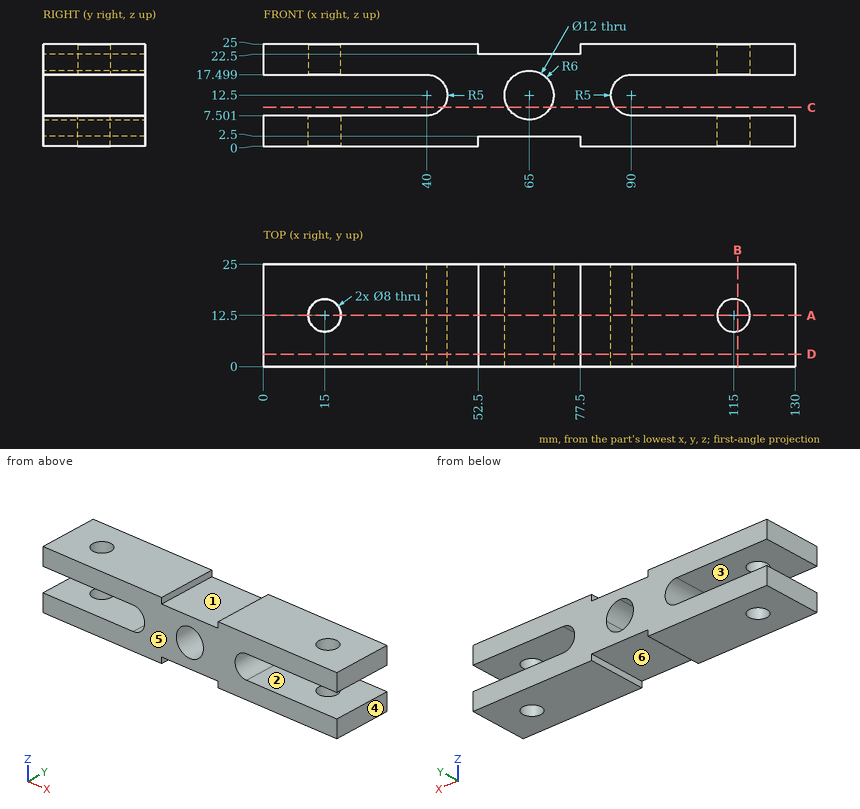
The drawing under review shows one solid part. Ordinate dimensions are in mm from its lowest x, y, z. A direction names the side the tool comes from. Coordinates: 2 decimals unless noted, no trailing zeros. Order: outer loops, then holes, each group sorted by start corner. A loop starts at its lowest first (then second) coordinate and runs counter-clockwise, first axis right, second up. Notation, with made-up numbers: (-2, 60.25) -> (4, 60.25) arc R36 cw to (4, 94.25) -> close; hole circle Ø7 at (45, 56). An arc over 180 degrees is marked (long way). Use CSV: the item, a comma, the result in double quotes. Start each with the question number.
Item 1: We need section D-D, the plane y = 3. Give the boundary of the cut face in (x, z) (1 decimal), then the cut area to 3 significant figures.
Item 2: Draft analysis for pull direction X (two halves, no side actions). For the marked faces 4, 5 and 6, state which applies: pulls with the +X half, pulls with the -X half, needs draft (parallel to the pull), parting line crosses it, or undercut.
Item 3: We need section C-C, the plane z = 9.5. Give the boundary of the cut face in (x, y).
Item 4: For the marked faces 1, 2 and 3, list the 3-axis set-ups (+Z, -Z, +X, -X, +Y, -Y) from which the entire face can be reached by the end or side of a thin tool; tool diameter is ignored.
Item 5: We need section A-A, the plane y = 12.5. Give the number of separate pieces and of enclosed holes in the cut face, then the cut area to 3 significant figures.
Item 6: We need section B-B, the plane x = 116. Give the boundary of the cut face in (y, z).
Item 7: Wall thickness on probe 1 along X at (y, z) = (23.5, 1); probe 2 along Y at (x, z) = (15, 5.25); probe 3 along Z at (x, y) = (28, 21): over which ranges is each line inside the solid? List them lowest first.
Item 8: Insertion check: pin 1 (5 mm diameter, centred on x = 115, y = 12.5, fed in from -Z). The pin has a flat end and moves straight along its axis. Give the tip position at first contact, or say it passes through.
Derived:
1,outline,"(0, 0) -> (52.5, 0) -> (52.5, 2.5) -> (77.5, 2.5) -> (77.5, 0) -> (130, 0) -> (130, 7.5) -> (90.1, 7.5) arc R5 cw (long way) to (90.1, 17.5) -> (130, 17.5) -> (130, 25) -> (77.5, 25) -> (77.5, 22.5) -> (52.5, 22.5) -> (52.5, 25) -> (0, 25) -> (0, 17.5) -> (39.9, 17.5) arc R5 cw (long way) to (39.9, 7.5) -> (0, 7.5) -> close; hole (65, 18.5) arc R6 ccw (long way) to (71, 12.5) arc R6 ccw to start"
1,area,"2,130 mm^2"
2,face 4,"pulls with the +X half"
2,face 5,"needs draft"
2,face 6,"undercut"
3,outline,"(44, 0) -> (59.8, 0) -> (59.8, 25) -> (44, 25) -> close; (70.2, 0) -> (86, 0) -> (86, 25) -> (70.2, 25) -> close"
4,face 1,"+Z, +Y, -Y"
4,face 2,"+X, +Y, -Y"
4,face 3,"-X, +Y, -Y"
5,separate pieces,"5"
5,enclosed holes,"1"
5,area,"1,890 mm^2"
6,outline,"(0, 0) -> (8.63, 0) -> (8.63, 7.5) -> (0, 7.5) -> close; (0, 17.5) -> (8.63, 17.5) -> (8.63, 25) -> (0, 25) -> close; (16.37, 0) -> (25, 0) -> (25, 7.5) -> (16.37, 7.5) -> close; (16.37, 17.5) -> (25, 17.5) -> (25, 25) -> (16.37, 25) -> close"
7,probe 1,"x = 0 to 52.5, 77.5 to 130"
7,probe 2,"y = 0 to 8.5, 16.5 to 25"
7,probe 3,"z = 0 to 7.5, 17.5 to 25"
8,pin 1,"passes through"
